Work out the finished part from the listing and answer in its coordinate system (mm). Round coordinates to 2 decimals unless told otherwise and drop trailing zeros. Order: outer loops, then holes, each group sorted by start corner. A loop starts at its lowest first (then second) coordinate and runs counter-clockwise, first axis right, second up. Notation, with made-up numbers: (-13, 26) - (19, 26) arc R17 cw to (19, 55) - close; hole circle Ø5 at (65, 76). An arc over 180 degrees is marked (long way). Put each result on its own line as item: value.
```python
from build123d import *

# Parameters (mm, degrees)
SKETCH1_R           = 4.7625
BOSS_EXTRUDE1_DEPTH = 12.7
SKETCH2_R           = 3.175
CUT_EXTRUDE1_DEPTH  = 26.4


with BuildPart() as part:
    # Sketch1 → Boss-Extrude1 (new body, symmetric)
    with BuildSketch(Plane(origin=(0, 0, 0), x_dir=(0, 0, -1), z_dir=(1, 0, 0))):
        with BuildLine():
            Line((-5.078713962, 127.1143), (-7.935490566, 0.17859375))
            ThreePointArc((-7.935490566, 0.17859375), (0, -7.9375), (7.935490566, 0.17859375))
            Line((7.935490566, 0.17859375), (5.078713962, 127.1143))
            ThreePointArc((5.078713962, 127.1143), (0, 132.08), (-5.078713962, 127.1143))
        make_face()
        Circle(SKETCH1_R, mode=Mode.SUBTRACT)
    extrude(amount=BOSS_EXTRUDE1_DEPTH, both=True)

    # Sketch2 → Cut-Extrude1 (cut, through all)
    with BuildSketch(Plane(origin=(12.7, 0, 0), x_dir=(0, 0, -1), z_dir=(1, 0, 0))):
        with Locations((0, 31.75)):
            Circle(SKETCH2_R)
        with Locations((0, 127)):
            Circle(SKETCH2_R)
    extrude(amount=-CUT_EXTRUDE1_DEPTH, mode=Mode.SUBTRACT)


solid = part.part
```
1) A cutting plane is placed at B-B on x = 10. Give the number of separate pieces and of enclosed holes in the cut face, then the cut area to 3 significant figures.
Findings below:
separate pieces: 1
enclosed holes: 3
area: 1,660 mm2
2) Straight lines are drawn through the part: L1, parallel to Y at x = -9.75, z = 0.25; L2, parallel to Y at x = -2.75, z = -0.5; L3, parallel to Z at x = -11, y = 110.5. For each, find the intervals that lie inside material, in ascending order. Write a range as from..to.
Findings below:
L1: y = -7.93..-4.76, 4.76..28.58, 34.92..123.83, 130.17..132.07
L2: y = -7.92..-4.74, 4.74..28.61, 34.89..123.86, 130.14..132.06
L3: z = -5.45..5.45
3) Given pin 1 Ø6 at (x, y) = (-9.5, 56.5) entering from +Z; pin 2 Ø8 at (x, z) = (3.5, 6) entering from +Y; pin 3 Ø12 at (x, y) = (-0.5, 57.5) entering from -Z, each flat-ended and moving along its own axis, determine where each tip first touches the part or whether it passes through.
Findings below:
pin 1: stops at z = 6.74
pin 2: stops at y = 131.67
pin 3: stops at z = -6.78
4) For a pull along Z with two mould halves and no side action, classify faces 1 (the flat face through (12.7, 63, 0)), 2 (the cylindrical face through (0.18, 130.15, 0.41)), 3 (the cylindrical face through (0.18, 132.08, -0.11)) as pulls with the +Z half, pulls with the -Z half, needs draft (parallel to the pull), parting line crosses it, or undercut.
Findings below:
face 1: needs draft
face 2: undercut
face 3: parting line crosses it
5) A cutting plane is placed at A-A on z = 0. Write down the section's boundary in (x, y) (1 decimal), then the cut area to 3 significant figures.
Findings below:
outline: (-12.7, -7.9) - (12.7, -7.9) - (12.7, -4.8) - (-12.7, -4.8) - close; (-12.7, 4.8) - (12.7, 4.8) - (12.7, 28.6) - (-12.7, 28.6) - close; (-12.7, 34.9) - (12.7, 34.9) - (12.7, 123.8) - (-12.7, 123.8) - close; (-12.7, 130.2) - (12.7, 130.2) - (12.7, 132.1) - (-12.7, 132.1) - close
area: 2,990 mm2
6) A cutting plane is placed at D-D on y = 31.75. Write down the section's boundary in (x, z) (3 decimals).
Findings below:
outline: (-12.7, -7.225) - (12.7, -7.225) - (12.7, -3.175) - (-12.7, -3.175) - close; (-12.7, 3.175) - (12.7, 3.175) - (12.7, 7.225) - (-12.7, 7.225) - close
7) A cutting plane is placed at C-C on y = 2.5. Write down the section's boundary in (x, z).
Findings below:
outline: (-12.7, -7.88) - (12.7, -7.88) - (12.7, -4.05) - (-12.7, -4.05) - close; (-12.7, 4.05) - (12.7, 4.05) - (12.7, 7.88) - (-12.7, 7.88) - close
